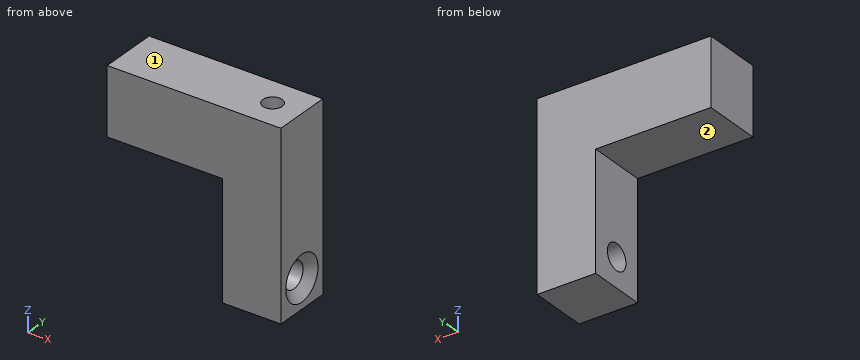
from build123d import *

# Parameters (mm, degrees)
SKETCH1_W                                          = 12.7
SKETCH1_H                                          = 40
BOSS_EXTRUDE1_DEPTH                                = 12.7
CSK_FOR_10_FLAT_HEAD_MACHINE_SCREW_100_D           = 5.6134
CSK_FOR_10_FLAT_HEAD_MACHINE_SCREW_100_DEPTH       = 12.7
CSK_FOR_10_FLAT_HEAD_MACHINE_SCREW_100_CSINK_D     = 9.779
CSK_FOR_10_FLAT_HEAD_MACHINE_SCREW_100_CSINK_ANGLE = 100
CSK_FOR_10_FLAT_HEAD_MACHINE_SCREW_100_TIP         = 1.686435499
TAP_DRILL_FOR_M5X0_8_TAP1_D                        = 4.2
TAP_DRILL_FOR_M5X0_8_TAP1_DEPTH                    = 12.7
TAP_DRILL_FOR_M5X0_8_TAP1_TIP                      = 1.2618073
SKETCH8_W                                          = 14.6
SKETCH8_H                                          = 12.7
BOSS_EXTRUDE2_DEPTH                                = 25


with BuildPart() as part:
    # Sketch1 → Boss-Extrude1 (new body)
    with BuildSketch(Plane(origin=(0, 0, 0), x_dir=(1, 0, 0), z_dir=(0, 1, 0))):
        with Locations((-5.02755102, -8.673469388)):
            Rectangle(SKETCH1_W, SKETCH1_H)
    extrude(amount=BOSS_EXTRUDE1_DEPTH)

    # CSK for #10 Flat Head Machine Screw (100)1
    with Locations(Plane(origin=(1.32244898, 0, 0), x_dir=(0, 0, -1), z_dir=(1, 0, 0))):
        with Locations((4.976530612, 6.35)):
            CounterSinkHole(CSK_FOR_10_FLAT_HEAD_MACHINE_SCREW_100_D / 2, CSK_FOR_10_FLAT_HEAD_MACHINE_SCREW_100_CSINK_D / 2, depth=CSK_FOR_10_FLAT_HEAD_MACHINE_SCREW_100_DEPTH, counter_sink_angle=CSK_FOR_10_FLAT_HEAD_MACHINE_SCREW_100_CSINK_ANGLE)
            with Locations((0, 0, -(CSK_FOR_10_FLAT_HEAD_MACHINE_SCREW_100_DEPTH + CSK_FOR_10_FLAT_HEAD_MACHINE_SCREW_100_TIP / 2))):  # 118° drill point
                Cone(0, CSK_FOR_10_FLAT_HEAD_MACHINE_SCREW_100_D / 2, CSK_FOR_10_FLAT_HEAD_MACHINE_SCREW_100_TIP, mode=Mode.SUBTRACT)

    # Tap Drill for M5x0.8 Tap1
    with Locations(Plane.XY.offset(28.673469388)):
        with Locations((-5.02755102, 6.35)):
            Hole(TAP_DRILL_FOR_M5X0_8_TAP1_D / 2, depth=TAP_DRILL_FOR_M5X0_8_TAP1_DEPTH)
            with Locations((0, 0, -(TAP_DRILL_FOR_M5X0_8_TAP1_DEPTH + TAP_DRILL_FOR_M5X0_8_TAP1_TIP / 2))):  # 118° drill point
                Cone(0, TAP_DRILL_FOR_M5X0_8_TAP1_D / 2, TAP_DRILL_FOR_M5X0_8_TAP1_TIP, mode=Mode.SUBTRACT)

    # Sketch8 → Boss-Extrude2 (add)
    with BuildSketch(Plane.ZY.offset(11.37755102)):
        with Locations((21.373469388, 6.35)):
            Rectangle(SKETCH8_W, SKETCH8_H)
    extrude(amount=BOSS_EXTRUDE2_DEPTH)


solid = part.part
Geometry check sheet. Reference: the model listing, model coordinates, mm. Face numbers are marked on the shaded views. A direction names the side the tool comes from. Round coordinates to 2 decimals unless told otherwise and drop trailing zeros. Order: outer loops, then holes, each group sorted by start corner. A loop starts at its lowest first (then second) coordinate and runs counter-clockwise, first axis right, second up. Notation, with made-up numbers: M 77.5,19 L 103.5,19 A15 cw 103.5,44 Z; hole C 23.25,-27.75 d10. An arc over 180 degrees is marked long. Answer in a Markdown table with one row per item. Add a question column.
Item 1: Sectioned sample at A-A, the plane z = 18. Enter the section's corners in (x, y), plus the area to 3 significant figures.
Item 2: Sectioned sample at B-B, the plane x = -9.5. Enter the section's corners in (y, z).
Item 3: Sectioned sample at D-D, the plane x = -34. Enter the section's corners in (y, z).
Item 4: Material ranges on L1, parallel to X at y = 6.35, z = 21.75; L2, parallel to Z at x = -22, y = 9.25; L3, parallel to X at y = 7, z = 5.5, recorded low to high. Write a range as [from, to].
Item 5: Depth check by flat-ended pin: pin 1 Ø6.5 at (y, z) = (4.5, 3.5) entering from -X; pin 2 Ø4 at (x, y) = (-19, 9.5) entering from -Z; pin 3 Ø3.5 at (y, z) = (6.35, -4.98) entering from +X. Enter the tip coordinate at first touch or a pass-through.
Item 6: Sectioned sample at C-C, the plane z = 3. Enter the section's corners in (x, y), plus the area to 3 significant figures.
Item 7: Set-up check for the marked faces 1 and 2: record each of +Z, -Z, +X, -X, +Y, -Y from which the full face is reachable in a straight line by a thin tool's end or side.
Filled in:
| question | item | result |
|---|---|---|
| 1 | outline | M -36.38,0 L 1.32,0 L 1.32,12.7 L -36.38,12.7 Z; hole C -5.03,6.35 d4.2 |
| 1 | area | 465 mm² |
| 2 | outline | M 0,-11.33 L 12.7,-11.33 L 12.7,28.67 L 0,28.67 Z; hole C 6.35,-4.98 d5.61 |
| 3 | outline | M 0,14.07 L 12.7,14.07 L 12.7,28.67 L 0,28.67 Z |
| 4 | L1 | x = [-36.38, -7.13], [-2.93, 1.32] |
| 4 | L2 | z = [14.07, 28.67] |
| 4 | L3 | x = [-11.38, 1.32] |
| 5 | pin 1 | stops at x = -11.38 |
| 5 | pin 2 | stops at z = 14.07 |
| 5 | pin 3 | passes through |
| 6 | outline | M -11.38,0 L 1.32,0 L 1.32,12.7 L -11.38,12.7 Z |
| 6 | area | 161 mm² |
| 7 | face 1 | +Z, +X, -X, +Y, -Y |
| 7 | face 2 | -Z, -X, +Y, -Y |
